from build123d import *

# Parameters (mm, degrees)
SKETCH1_R           = 2.285
SKETCH1_R_2         = 1.27
BOSS_EXTRUDE1_DEPTH = 3.048
BOSS_EXTRUDE2_DEPTH = 3.048
CIRPATTERN1_COUNT   = 18
SKETCH3_R           = 1.75
SKETCH3_R_2         = 1.27
BOSS_EXTRUDE3_DEPTH = 2.54


with BuildPart() as part:
    # Sketch1 → Boss-Extrude1 (new body)
    with BuildSketch(Plane(origin=(0, 0, 0), x_dir=(1, 0, 0), z_dir=(0, 1, 0))):
        Circle(SKETCH1_R)
        Circle(SKETCH1_R_2, mode=Mode.SUBTRACT)
    extrude(amount=BOSS_EXTRUDE1_DEPTH)

    # Sketch2 → Boss-Extrude2 (add)
    with BuildSketch(Plane(origin=(0, 3.048, 0), x_dir=(1, 0, 0), z_dir=(0, 1, 0))):
        with BuildLine():
            Line((-0.127, 2.792943956), (0.127, 2.792943956))
            Line((0.127, 2.792943956), (0.38, 2.253139456))
            ThreePointArc((0.38, 2.253139456), (0, 2.285), (-0.38, 2.253139456))
            Line((-0.38, 2.253139456), (-0.127, 2.792943956))
        make_face()
    boss_extrude2 = extrude(amount=-BOSS_EXTRUDE2_DEPTH)

    # CirPattern1: Boss-Extrude2 ×18 about axis
    cirpattern1_axis = Axis((0, 0, 0), (0, 1, 0))
    for i in range(1, CIRPATTERN1_COUNT):
        add(boss_extrude2.rotate(cirpattern1_axis, i * 360 / CIRPATTERN1_COUNT))

    # Sketch3 → Boss-Extrude3 (add)
    with BuildSketch(Plane.XZ):
        Circle(SKETCH3_R)
        Circle(SKETCH3_R_2, mode=Mode.SUBTRACT)
    extrude(amount=BOSS_EXTRUDE3_DEPTH)


solid = part.part
Can you work these out from the model? Positions are in its coordinate system, mm. Coordinates: 2 decimals unless noted, no trailing zeros. Order: outer loops, then holes, each group sorted by start corner. A loop starts at its lowest first (then second) coordinate and runs counter-clockwise, first axis right, second up. Notation, with made-up numbers: (72, 48.25) - (89, 48.25) arc R14 cw to (89, 55.25) - close; hole circle Ø4 at (11, 69.5). An arc over 180 degrees is marked (long way). Answer as a JSON object with one key per item and string values. Group by question number.
Q1. Will this pin go through, and if not, where does the flat tip stop? P1, Ø3, axis at x = 0, z = 0, coming from the +Y side.
Q2. Imagine slicing it at B-B (z = 1). Please give me the cut outline in (x, y), and give its area (3 significant figures).
Q3. I need wall thicknesses on line 1 (X direction, y = -2.2, z = -0.05); line 2 (Z direction, x = 0, y = 0.4). Which ranges of each line are inside material? Lowest first, please. Write a range as from..to.
Q4. Imagine slicing it at D-D (y = -0.4). Please give me the cut outline in (x, z), and give its area (3 significant figures).
Q5. We'd pull the mould along Z, two halves only. Please class faces 1 (the face through (1.617, -1.252, -0.67)), 2 (the face through (-0.17, 0.29, 1.26)), 3 (the face through (-2, 0, -1)): +Z half, -Z half, draft (parallel to the pull), parting line (faces both ways), or undercut.
Q6. Imagine slicing it at C-C (z = 2.4). Please give me the cut outline in (x, y).
Q7. Imagine slicing it at A-A (x = 0). Please give me the cut outline in (y, z).
Determined:
{
 "1": {"P1": "stops at y = 3.05"},
 "2": {"outline": "(-2.28, 0) - (-1.44, 0) - (-1.44, -2.54) - (-0.78, -2.54) - (-0.78, 3.05) - (-2.28, 3.05) - close; (0.78, -2.54) - (1.44, -2.54) - (1.44, 0) - (2.28, 0) - (2.28, 3.05) - (0.78, 3.05) - close", "area": "12.5 mm2"},
 "3": {"line 1": "x = -1.75..-1.27, 1.27..1.75", "line 2": "z = -2.79..-1.27, 1.27..2.79"},
 "4": {"outline": "circle Ø3.5 at (0, 0); hole circle Ø2.54 at (0, 0)", "area": "4.55 mm2"},
 "5": {"face 1": "parting line", "face 2": "undercut", "face 3": "draft"},
 "6": {"outline": "(-1.09, 0) - (-0.57, 0) - (-0.57, 3.05) - (-1.09, 3.05) - close; (-0.31, 0) - (0.31, 0) - (0.31, 3.05) - (-0.31, 3.05) - close; (0.57, 0) - (1.09, 0) - (1.09, 3.05) - (0.57, 3.05) - close"},
 "7": {"outline": "(-2.54, -1.75) - (0, -1.75) - (0, -2.79) - (3.05, -2.79) - (3.05, -1.27) - (-2.54, -1.27) - close; (-2.54, 1.27) - (3.05, 1.27) - (3.05, 2.79) - (0, 2.79) - (0, 1.75) - (-2.54, 1.75) - close"}
}
